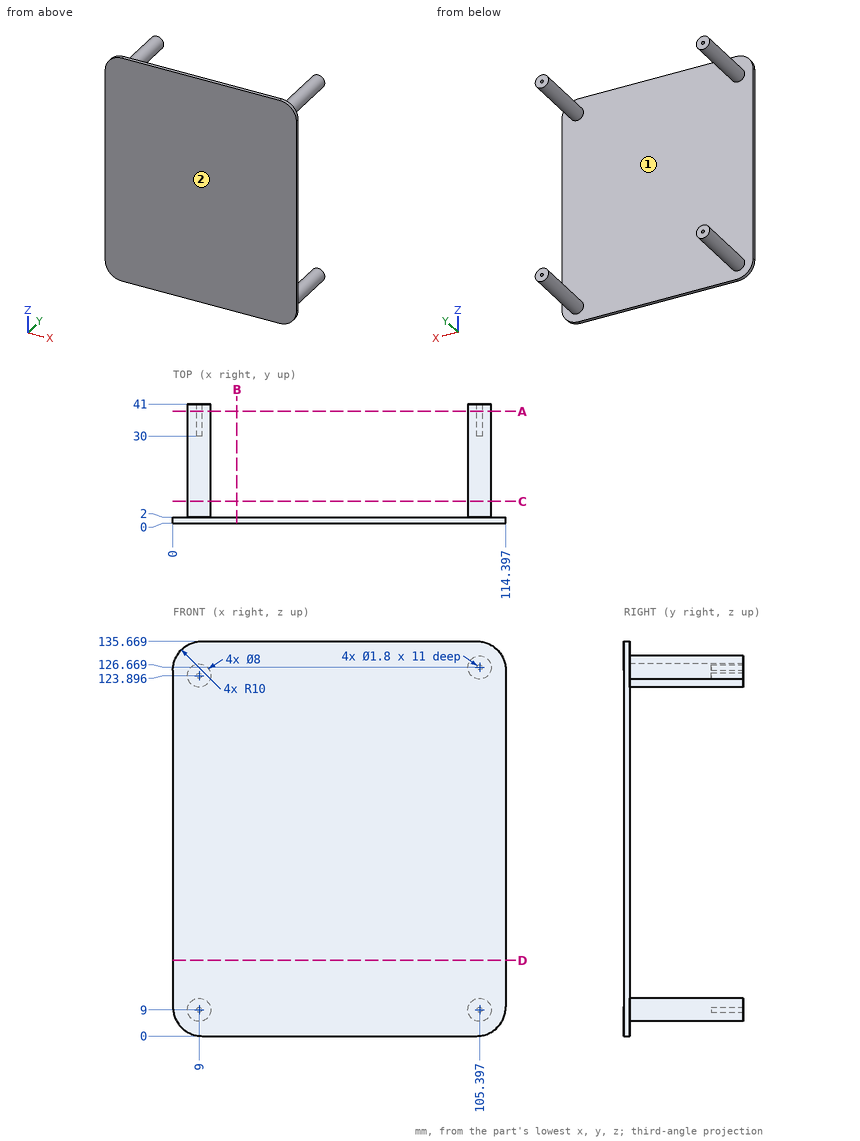
Verification items for this drawing (mm, ordinates from the low corner). Round coordinates to 2 decimals unless told otherwise and drop trailing zeros. Order: outer loops, then holes, each group sorted by start corner. A loop starts at its lowest first (then second) coordinate and runs counter-clockwise, first axis right, second up. Notation, with made-up numbers: (-10, 32.25) - (4, 32.25) arc R13 cw to (4, 48.25) - close; hole circle Ø5 at (15, -6.75). An arc over 180 degrees is marked (long way). Use CSV: the item, a comma, the result in double quotes. Start each with the question number.
1) Thickness scan on L1, parallel to Z at x = 9, y = 35; L2, parallel to Y at x = 61.5, z = 114. Record the ranges inside material, lowest first.
2) Go/stop test with flat-tipped pins: P1, Ø3, axis at y = 16.5, z = 14, coming from the -X side (1 decimal); P2, Ø10, axis at x = 34, z = 59.5, coming from the +Y side; P3, Ø0.5, axis at x = 105, z = 9, coming from the +Y side. Record where each tip stops, or that it passes through.
3) Mould release check, pull along Z, two halves, no side actions. Record for the marked faces 1 and 2: +Z half, -Z half, draft (parallel to the pull), parting line (faces both ways), or undercut.
4) Section check D-D, the plane z = 26. Record the cut outline in (x, y).
5) Section check C-C, the plane y = 7.5. Record the cut outline in (x, z), plus the area to 3 significant figures.
6) Section check A-A, the plane y = 38.5. Record the cut outline in (x, z), plus the area to 3 significant figures.
7) Section check B-B, the plane x = 22. Record the cut outline in (y, z).
Answers:
1,L1,"z = 5 to 8.1, 9.9 to 13, 119.9 to 123, 124.8 to 127.9"
1,L2,"y = 0 to 2"
2,P1,"stops at x = 7.1"
2,P2,"stops at y = 2"
2,P3,"stops at y = 30"
3,face 1,"undercut"
3,face 2,"draft"
4,outline,"(0, 0) - (114.4, 0) - (114.4, 2) - (0, 2) - close"
5,outline,"circle Ø8 at (9, 9); circle Ø8 at (9, 123.9); circle Ø8 at (105.4, 9); circle Ø8 at (105.4, 126.67)"
5,area,"201 mm²"
6,outline,"circle Ø8 at (9, 9); circle Ø8 at (9, 123.9); circle Ø8 at (105.4, 9); circle Ø8 at (105.4, 126.67); hole circle Ø1.8 at (9, 9); hole circle Ø1.8 at (9, 123.9); hole circle Ø1.8 at (105.4, 9); hole circle Ø1.8 at (105.4, 126.67)"
6,area,"191 mm²"
7,outline,"(0, 0) - (2, 0) - (2, 135.67) - (0, 135.67) - close"
